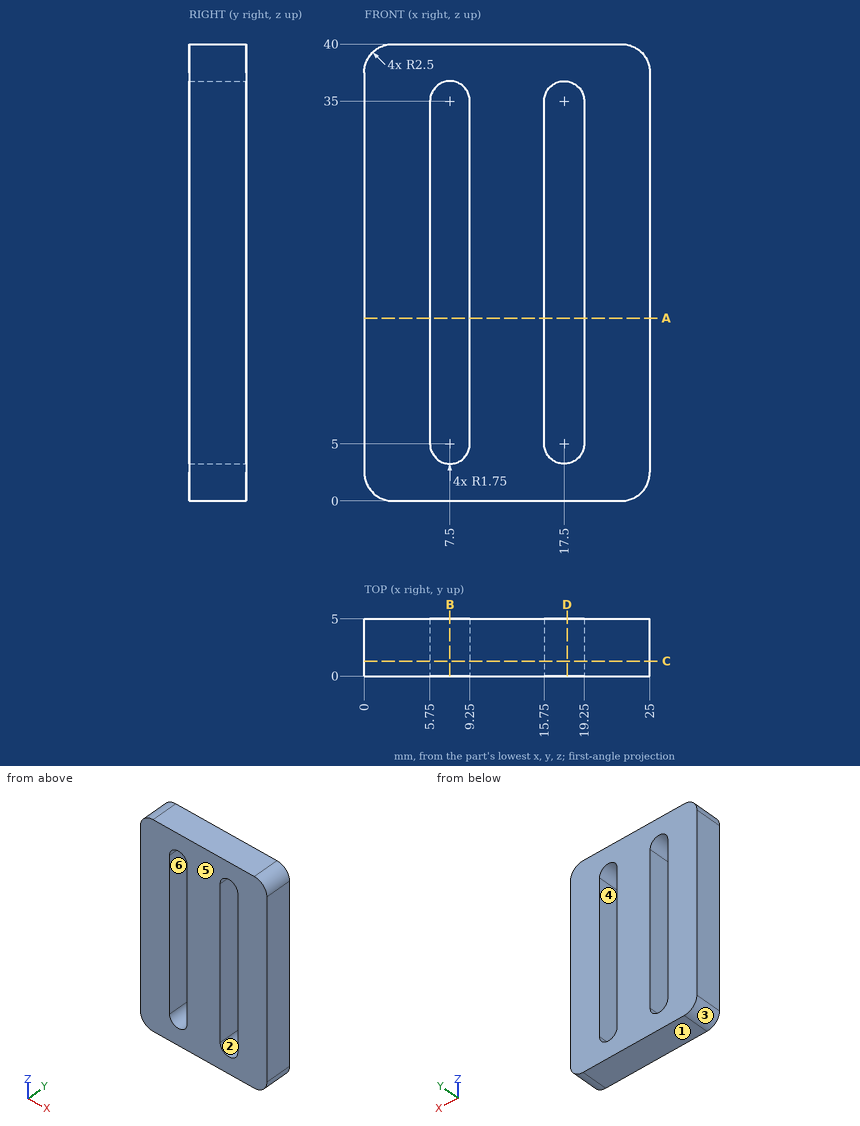
Could you check a few things on this drawing? It's one solid part, dimensions in mm from its lowest x, y, z. A direction names the side the tool comes from. Round coordinates to 2 decimals unless told otherwise and drop trailing zeros. Write each loop counter-clockwise with the first axis right and the second up, starting at its lowest first coordinate (ties: lowest second). Pieces come first, ordered by that corner, then holes.
Q1. Which directions (+Z, -Z, +X, -X, +Y, -Y) give clear straight access to the entire face, cutting with the end or side of a thin tool? Please do the marked faces 5 and 6.
Q2. If we section it at C-C on y = 1.3: Write out the boundary of the cut face in (x, z).
Q3. If we section it at B-B on x = 7.5: Write out the boundary of the cut face in (y, z).
Q4. If we section it at D-D on x = 17.75: Write out the boundary of the cut face in (y, z).
Q5. If we mould it in two halves opening along X, with no side actions, what happens to the marked faces 1, 2, 3 and 4? For each: +X half, -X half, draft (parallel to the pull), parting line (faces both ways), or undercut.
Q6. If we section it at A-A on z = 16: Write out the boundary of the cut face in (x, y).
Q7. Please list where these lines run through material, in increasing order: probe 1 along X at (y, z) = (1, 6.5); probe 2 along Z at (x, y) = (17.5, 0.2); probe 3 along X at (y, z) = (2.3, 36).
Answer below:
1. face 5: +Z, -Z, +X, -X, -Y
1. face 6: +Y, -Y
2. outline: (0, 2.5) arc R2.5 ccw to (2.5, 0) - (22.5, 0) arc R2.5 ccw to (25, 2.5) - (25, 37.5) arc R2.5 ccw to (22.5, 40) - (2.5, 40) arc R2.5 ccw to (0, 37.5) - close; hole (5.75, 5) arc R1.75 ccw to (9.25, 5) - (9.25, 35) arc R1.75 ccw to (5.75, 35) - close; hole (15.75, 5) arc R1.75 ccw to (19.25, 5) - (19.25, 35) arc R1.75 ccw to (15.75, 35) - close
3. outline: (0, 0) - (5, 0) - (5, 3.25) - (0, 3.25) - close; (0, 36.75) - (5, 36.75) - (5, 40) - (0, 40) - close
4. outline: (0, 0) - (5, 0) - (5, 3.27) - (0, 3.27) - close; (0, 36.73) - (5, 36.73) - (5, 40) - (0, 40) - close
5. face 1: draft
5. face 2: undercut
5. face 3: -X half
5. face 4: undercut
6. outline: (0, 0) - (5.75, 0) - (5.75, 5) - (0, 5) - close; (9.25, 0) - (15.75, 0) - (15.75, 5) - (9.25, 5) - close; (19.25, 0) - (25, 0) - (25, 5) - (19.25, 5) - close
7. probe 1: x = 0 to 5.75, 9.25 to 15.75, 19.25 to 25
7. probe 2: z = 0 to 3.25, 36.75 to 40
7. probe 3: x = 0 to 6.06, 8.94 to 16.06, 18.94 to 25
